Source: CAD feature listing. Evaluate the final solid. Frame: model axes, mm. Give positions to 0.01 mm unless a question says otherwise; leave off trailing zeros. Loops run counter-clockwise (first coordinate to the right, second up) from the corner with the lowest first, then second, coordinate; pieces in that order, holes last.
from build123d import *

# Parameters (mm, degrees)
BOSS_EXTRUDE1_DEPTH   = 5
F_8_0MM_DOWEL_HOLE1_D = 8


with BuildPart() as part:
    # Sketch1 → Boss-Extrude1 (new, symmetric)
    with BuildSketch(Plane.XY):
        with BuildLine():
            Line((-70, 10), (70, 10))
            ThreePointArc((70, 10), (80, 0), (70, -10))
            Line((70, -10), (-70, -10))
            ThreePointArc((-70, -10), (-80, 0), (-70, 10))
        make_face()
    extrude(amount=BOSS_EXTRUDE1_DEPTH, both=True)

    # Ø8.0mm Dowel Hole1 (through all)
    with Locations(Plane.XY.offset(5)):
        with Locations((-70, 0), (70, 0)):
            Hole(F_8_0MM_DOWEL_HOLE1_D / 2)


solid = part.part
1) Pull-direction query (X, two-part tool) for faces 1 (the cylindrical face through (66.305, -1.532, -0.07)), 2 (the flat face through (1, -10, 0)), 3 (the cylindrical face through (-80, 0, 0)), 4 (the cylindrical face through (-73.695, -1.532, -0.07)); classes: released by +X, released by -X, zero draft, split by the parting line, or undercut.
Checks:
face 1: undercut
face 2: zero draft
face 3: released by -X
face 4: undercut
2) Contact query for a flat-ended pin moving along its axis: P1, Ø1, axis at y = -4.5, z = 0.5, coming from the +X side. Output: stop coordinate, or through.
Checks:
P1: stops at x = 79.17
3) Cut plane B-B (z = 3.5). Return loops of the section in (x, y).
Checks:
outline: (-70, -10) - (70, -10) arc R10 ccw to (70, 10) - (-70, 10) arc R10 ccw to start; hole circle Ø8 at (-70, 0); hole circle Ø8 at (70, 0)
4) Cut plane A-A (y = 0). Return loops of the section in (x, z).
Checks:
outline: (-80, -5) - (-74, -5) - (-74, 5) - (-80, 5) - close; (-66, -5) - (66, -5) - (66, 5) - (-66, 5) - close; (74, -5) - (80, -5) - (80, 5) - (74, 5) - close
5) Ray query, probe 1 along Y at (x, z) = (70, 1.25); probe 2 along X at (y, z) = (1.25, 3.5); probe 3 along X at (y, z) = (-1.5, -2.5). Return the intervals inside material, ascending.
Checks:
probe 1: y = -10 to -4, 4 to 10
probe 2: x = -79.92 to -73.8, -66.2 to 66.2, 73.8 to 79.92
probe 3: x = -79.89 to -73.71, -66.29 to 66.29, 73.71 to 79.89
6) Cut plane C-C (y = 8.5). Return loops of the section in (x, z), and give its area (3 significant figures).
Checks:
outline: (-75.27, -5) - (75.27, -5) - (75.27, 5) - (-75.27, 5) - close
area: 1,510 mm2
